```python
from build123d import *

# Parameters (mm, degrees)
F0_W     = 1828.8
F0_H     = 609.6
F1_DEPTH = 101.6
F2_W     = 1828.8
F2_H     = 508
F3_DEPTH = 88.9
F4_R     = 25.4


with BuildPart() as f1:
    # F0 (on Front) → F1 (new body)
    with BuildSketch(Plane.XZ):
        with Locations((0, -304.8)):
            Rectangle(F0_W, F0_H)
    extrude(amount=F1_DEPTH)

    # F2 (on face) → F3 (cut)
    with BuildSketch(Plane(origin=(0, 0, 0), x_dir=(-1, 0, 0), z_dir=(0, 1, 0))):
        with Locations((0, -355.6)):
            Rectangle(F2_W, F2_H)
    extrude(amount=-F3_DEPTH, mode=Mode.SUBTRACT)

    # F4
    f4_edges = [f1.edges().sort_by_distance(p)[0] for p in [
        (0, -101.6, 0),
    ]]
    fillet(f4_edges, radius=F4_R)


solid = f1.part
```
Could you check a few things on this model? Use its own coordinates, in mm. A direction names the side the tool comes from. Coordinates: 2 decimals unless noted, no trailing zeros. Loops run counter-clockwise (first coordinate to the right, second up) from the corner with the lowest first, then second, coordinate; pieces in that order, holes last.
1) Please list where these lines run through material, in increasing order: line 1 along Y through (x, z) = (-816, -237.5); line 2 along Z through (x, y) = (-544.5, -44); line 3 along Z through (x, y) = (-557, -90).
Reported:
line 1: y = -101.6 to -88.9
line 2: z = -101.6 to 0
line 3: z = -609.6 to -4.08
2) Will these pins go through, and if not, where does the flat tip stop? pin 1 Ø5 at (x, z) = (-45.5, -131.5) entering from +Y; pin 2 Ø1 at (x, y) = (540, -85.5) entering from -Z.
Reported:
pin 1: stops at y = -88.9
pin 2: stops at z = -101.6
3) Imagine slicing it at A-A (x = -746). List the corners of the cut face in (y, z) for me, and give its area (3 significant figures).
Reported:
outline: (-101.6, -609.6) - (-88.9, -609.6) - (-88.9, -101.6) - (0, -101.6) - (0, 0) - (-76.2, 0) arc R25.4 ccw to (-101.6, -25.4) - close
area: 16,600 mm2
4) Imagine slicing it at C-C (z = -398). List the corners of the cut face in (x, y) for me, and give its area (3 significant figures).
Reported:
outline: (-914.4, -101.6) - (914.4, -101.6) - (914.4, -88.9) - (-914.4, -88.9) - close
area: 23,200 mm2
5) Imagine slicing it at B-B (y = -23). List the corners of the cut face in (x, z) for me, and give its area (3 significant figures).
Reported:
outline: (-914.4, -101.6) - (914.4, -101.6) - (914.4, 0) - (-914.4, 0) - close
area: 186,000 mm2
6) Which directions (+Z, -Z, +X, -X, +Y, -Y) give clear straight access to the entire face, cutting with the end or side of a thin tool? Please do faces 1 (the face through (13, -44, -101.6)), 2 (the face through (-13, -101.6, -313)).
Reported:
face 1: -Z, +X, -X, +Y
face 2: +Z, -Z, +X, -X, -Y
